Autodesk Fusion 360 part; units mm, degrees
sketch "Base Sketch" plane through (0, 0, 0) normal (0, 0, 1) x (1, 0, 0)
  line L0 (0, 0) -> (106, 0)
  line L1 (106, 0) -> (106, 106)
  line L2 (106, 106) -> (0, 106)
  line L3 (0, 106) -> (0, 0)
  line L4 (19.5, 106) -> (86.5, 106)
  line L5 (86.5, 106) -> (86.5, 0)
  line L6 (86.5, 0) -> (19.5, 0)
  line L7 (19.5, 0) -> (19.5, 106)
  line L8 (21.5, 3) -> (84.5, 3)
  line L9 (84.5, 3) -> (84.5, 104)
  line L10 (84.5, 104) -> (21.5, 104)
  line L11 (21.5, 104) -> (21.5, 3)
  circle A0 centre (23, 7) radius 3
  circle A1 centre (23, 7) radius 0.9
  circle A2 centre (83, 7) radius 0.9
  circle A3 centre (83, 7) radius 3
  circle A4 centre (83, 99) radius 0.9
  circle A5 centre (83, 99) radius 3
  circle A6 centre (23, 99) radius 0.9
  circle A7 centre (23, 99) radius 3
  line L12 (80, 106) -> (80, 104)
  line L13 (52, 106) -> (52, 104)
  line L14 (37, 106) -> (37, 104)
  line L15 (86.5, 5) -> (106, 5)
  line L16 (106, 5) -> (106, 0)
  line L17 (106, 0) -> (86.5, 0)
  line L18 (86.5, 0) -> (86.5, 5)
  line L19 (0, 5) -> (19.5, 5)
  line L20 (19.5, 5) -> (19.5, 0)
  line L21 (19.5, 0) -> (0, 0)
  line L22 (0, 0) -> (0, 5)
  line L23 (86.5, 106) -> (106, 106)
  line L24 (106, 106) -> (106, 98.5)
  line L25 (106, 98.5) -> (86.5, 98.5)
  line L26 (86.5, 98.5) -> (86.5, 106)
  line L27 (0, 106) -> (19.5, 106)
  line L28 (19.5, 106) -> (19.5, 98.5)
  line L29 (19.5, 98.5) -> (0, 98.5)
  line L30 (0, 98.5) -> (0, 106)
  line L31 (106, 76.5) -> (86.5, 76.5)
  line L32 (86.5, 76.5) -> (86.5, 80)
  line L33 (86.5, 80) -> (106, 80)
  line L34 (106, 80) -> (106, 76.5)
  line L35 (0, 76.5) -> (19.5, 76.5)
  line L36 (19.5, 76.5) -> (19.5, 80)
  line L37 (19.5, 80) -> (0, 80)
  line L38 (0, 80) -> (0, 76.5)
  line L39 (63.5, 104) -> (80, 104)
  line L40 (80, 104) -> (80, 81)
  line L41 (36.5, 8) -> (71.5, 8)
  line L42 (71.5, 52) -> (83, 52)
  line L43 (83, 52) -> (83, 9.5)
  line L44 (83, 9.5) -> (71.5, 9.5)
  line L45 (71.5, 9.5) -> (71.5, 52)
  line L46 (62, 106) -> (62, 104)
  line L47 (62, 104) -> (62, 81)
  line L48 (36.5, 80) -> (71.5, 80)
  line L49 (36.5, 80) -> (36.5, 8)
  line L50 (71.5, 8) -> (71.5, 80)
  line L51 (62, 81) -> (80, 81)
  line L52 (36.5, 80) -> (62, 80)
  line L53 (62, 80) -> (62, 82)
  line L54 (62, 82) -> (36.5, 82)
  line L55 (36.5, 82) -> (36.5, 80)
  line L56 (62, 106) -> (60, 106)
  line L57 (60, 106) -> (60, 82)
  line L58 (60, 82) -> (62, 82)
  line L59 (62, 82) -> (62, 106)
  line L60 (80, 81) -> (82, 81)
  line L61 (82, 81) -> (82, 106)
  line L62 (82, 106) -> (80, 106)
  line L63 (80, 106) -> (80, 81)
  line L64 (82, 81) -> (71.5, 81)
  line L65 (71.5, 81) -> (71.5, 79)
  line L66 (71.5, 79) -> (82, 79)
  line L67 (82, 79) -> (82, 81)
  line L68 (71.5, 79) -> (73.5, 79)
  line L69 (73.5, 79) -> (73.5, 52)
  line L70 (73.5, 52) -> (71.5, 52)
  line L71 (71.5, 52) -> (71.5, 79)
  line L72 (36.5, 82) -> (34.5, 82)
  line L73 (34.5, 82) -> (34.5, 6)
  line L74 (34.5, 6) -> (36.5, 6)
  line L75 (36.5, 6) -> (36.5, 82)
  line L76 (36.5, 6) -> (71.5, 6)
  line L77 (71.5, 6) -> (71.5, 8)
  line L78 (71.5, 8) -> (36.5, 8)
  line L79 (36.5, 8) -> (36.5, 6)
  line L80 (71.5, 6) -> (72.5, 6)
  line L81 (72.5, 6) -> (72.5, 52)
  line L82 (72.5, 52) -> (71.5, 52)
  line L83 (71.5, 52) -> (71.5, 6)
  line L84 (62, 81) -> (73.5, 81)
  line L85 (73.5, 81) -> (73.5, 82)
  line L86 (73.5, 82) -> (62, 82)
  line L87 (62, 82) -> (62, 81)
  line L88 (73.5, 81) -> (73.5, 79)
  line L89 (51, 55) -> (59, 55)
  line L90 (59, 55) -> (59, 51)
  line L91 (59, 51) -> (51, 51)
  line L92 (51, 51) -> (51, 55)
  circle A8 centre (60.5, 22.5) radius 2
  circle A9 centre (40, 21.5) radius 1.5
  circle A10 centre (40, 13.5) radius 1.5
  dimension "d1" = 106
  dimension "d2" = 106
  dimension "d4" = 67
  dimension "d5" = 19.5
  dimension "d6" = 63
  dimension "d8" = 2
  dimension "d9" = 3
  dimension "d10" = 6
  dimension "d12" = 6
  dimension "d13" = 6
  dimension "d14" = 6
  dimension "d15" = 23
  dimension "d16" = 23
  dimension "d17" = 23
  dimension "d18" = 23
  dimension "d19" = 7
  dimension "d20" = 7
  dimension "d21" = 7
  dimension "d22" = 7
  dimension "d24" = 2
  dimension "d25" = 6.5
  dimension "d28" = 15
  dimension "d35" = 5
  dimension "d36" = 5
  dimension "d37" = 7.5
  dimension "d38" = 7.5
  dimension "d39" = 3.5
  dimension "d40" = 26
  dimension "d41" = 3.5
  dimension "d42" = 26
  dimension "d45" = 8
  dimension "d48" = 42.5
  dimension "d49" = 9.5
  dimension "d60" = 10
  dimension "d62" = 18
  dimension "d63" = 1.8
  dimension "d64" = 1.8
  dimension "d65" = 1.8
  dimension "d66" = 1.8
  dimension "d68" = 72
  dimension "d69" = 25
  dimension "d70" = 35
  dimension "d71" = 2
  dimension "d72" = 2
  dimension "d73" = 2
  dimension "d74" = 2
  dimension "d75" = 2
  dimension "d76" = 11.5
  dimension "d77" = 2
  dimension "d78" = 2
  dimension "d87" = 1
  dimension "d88" = 25.5
  dimension "d89" = 44
  dimension "d90" = 36.5
  dimension "d94" = 1
  dimension "d95" = 11.5
  dimension "d96" = 8
  dimension "d97" = 4
  dimension "d98" = 25
  dimension "d99" = 14.5
  dimension "d100" = 4
  dimension "d101" = 3
  dimension "d102" = 3
  dimension "d103" = 5.5
  dimension "d104" = 13.5
  dimension "d105" = 3.5
  dimension "d106" = 3.5
  dimension "d107" = 14.5
  dimension "d108" = 24
extrude "Extrude1" add sketch "Base Sketch" against normal blind 9 contours L0 L3 L7 L19 L20 L21 L22 | L0 L2 L4 L5 L6 L7 L8 L9 L10 L11 A0 A3 A5 A7 L14 L18 L20 L26 L28 L32 L36 L61 | L0 L1 L5 L15 L16 L17 L18 | L3 L7 L35 L36 L37 L38 | L1 L5 L31 L32 L33 L34 | L2 L3 L7 L27 L28 L29 L30 | L1 L2 L5 L23 L24 L25 L26 | L2 L4 L10 L12 L61 L62 L63 | A5 L61 | L9 A5 L61 | L11 A7 | L11 A7 | L9 A5 | L11 A0 | L11 A0 | L9 A3 | L9 A3 L43 L44 | A3 L43 L44 makes body 1
extrude "Extrude2" add sketch "Base Sketch" against normal blind 6 contours L2 L4 L10 L13 L14 bodies 1
extrude "Extrude3" add sketch "Base Sketch" against normal blind 5 contours L2 L4 L10 L13 L57 | L2 L4 L10 L46 L56 L57 L59 bodies 1
extrude "Extrude4" add sketch "Base Sketch" against normal blind 2 separate body contours L0 L2 L4 L5 L6 L7 L8 L9 L10 L11 A0 A3 A5 A7 L14 L18 L20 L26 L28 L32 L36 L61 | L2 L4 L10 L13 L14 | L2 L4 L10 L12 L61 L62 L63 | L2 L4 L10 L13 L57 | L8 L9 L10 L11 A0 A3 A7 L44 L54 L57 L72 L73 L74 L76 L80 L81 | L2 L4 L10 L12 L39 L46 L59 L63 | L9 L10 A5 L61 | L2 L4 L10 L46 L56 L57 L59 | A5 L61 | L9 A5 L61 | L10 L47 L54 L57 L58 L59 | L11 A7 | L11 A7 | A5 L40 L60 L61 L63 L64 | L9 A5 | L9 A3 A5 L42 L43 L61 L66 L67 L69 | L47 L48 L52 L53 L54 L55 L58 L75 L87 | L51 L60 L64 L66 L67 L88 | L49 L55 L72 L73 L74 L75 L79 | L11 A0 | L11 A0 | L48 L51 L53 L65 L84 | L50 L51 L64 L65 L66 L68 L84 L88 | L9 A3 | L9 A3 L43 L44 | L42 L50 L66 L68 L69 L70 L71 L82 | A3 L43 L44 | L41 L75 L76 L77 L78 L79 L83 | L44 L50 L77 L80 L81 L83 | A1 | A2 | A4 | A6 makes body 2
chamfer "Chamfer1" distance 8 angle 45 1 edges at (106, 102.25, 0) on bodies 1
chamfer "Chamfer2" distance 8 angle 45 1 edges at (106, 78.25, 0) on bodies 1
chamfer "Chamfer3" distance 8 angle 45 1 edges at (106, 2.5, 0) on bodies 1
chamfer "Chamfer4" distance 8 angle 45 1 edges at (0, 102.25, 0) on bodies 1
chamfer "Chamfer5" distance 8 angle 45 1 edges at (0, 78.25, 0) on bodies 1
chamfer "Chamfer6" distance 8 angle 45 1 edges at (0, 2.5, 0) on bodies 1
extrude "Extrude5" add sketch "Base Sketch" along normal blind 7 contours L47 L48 L52 L53 L54 L55 L58 L75 L87 | L49 L55 L72 L73 L74 L75 L79 | L48 L51 L53 L65 L84 | L50 L51 L64 L65 L66 L68 L84 L88 | L42 L50 L66 L68 L69 L70 L71 L82 | L41 L75 L76 L77 L78 L79 L83 | L44 L50 L77 L80 L81 L83 | L42 L44 L45 L50 L70 L81 L82 L83 bodies 2
extrude "Extrude6" add sketch "Base Sketch" along normal blind 2 from surface at 7 separate body contours L47 L48 L52 L53 L54 L55 L58 L75 L87 | L49 L55 L72 L73 L74 L75 L79 | L48 L51 L53 L65 L84 | L50 L51 L64 L65 L66 L68 L84 L88 | L41 L45 L48 L49 L50 L52 L65 L71 L75 L78 L83 | L42 L50 L66 L68 L69 L70 L71 L82 | L41 L75 L76 L77 L78 L79 L83 | L44 L50 L77 L80 L81 L83 | L42 L44 L45 L50 L70 L81 L82 L83 makes body 3
extrude "Extrude7" add sketch "Base Sketch" along normal blind 5.5 contours L2 L4 L10 L12 L61 L62 L63 | L10 A5 L40 L61 L63 | L2 L4 L10 L46 L56 L57 L59 | A5 L61 | L10 L47 L54 L57 L58 L59 | A5 L40 L60 L61 L63 L64 | L51 L60 L64 L66 L67 L88 bodies 2 1
extrude "Extrude8" add sketch "Base Sketch" along normal blind 2 from surface at 5.5 separate body contours L2 L4 L10 L12 L61 L62 L63 | L2 L4 L10 L12 L39 L46 L59 L63 | L10 A5 L40 L61 L63 | L2 L4 L10 L46 L56 L57 L59 | L10 L39 L40 L47 L51 L59 L63 L64 L85 L86 | A5 L61 | L10 L47 L54 L57 L58 L59 | A5 L40 L60 L61 L63 L64 | L51 L60 L64 L66 L67 L88 makes body 4
extrude "Extrude9" add sketch "Base Sketch" along normal blind 3.5 from surface at 5.5 contours L47 L51 L53 L64 L84 L85 L86 L87 bodies 2 3 4
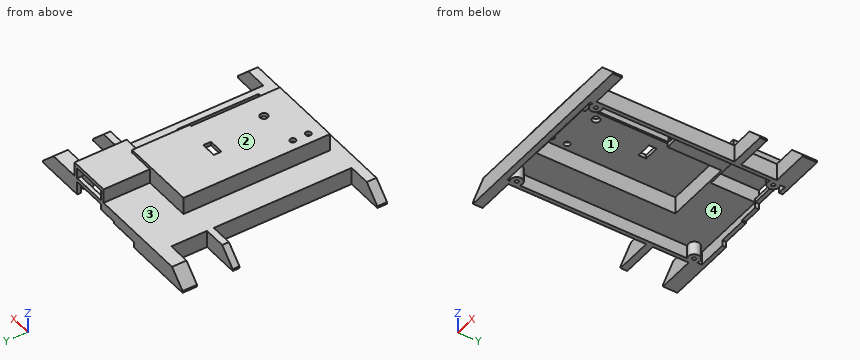
Design review of the part built by this model. Coordinates are the model's own, in mm. Face numbers are marked on the shaded views. A direction names the side the tool comes from. Coordinates: 2 decimals unless noted, no trailing zeros. Write each loop counter-clockwise with the first axis right and the second up, starting at its lowest first coordinate (ties: lowest second). Pieces come first, ordered by that corner, then holes. Notation, with made-up numbers: (-32.75, 58) - (-28.75, 58) arc R26 cw to (-28.75, 74) - close; hole circle Ø9 at (80.5, -40). An arc over 180 degrees is marked (long way). Use one line per item in the form item = value.
Q1. The part is to be moulded in two halves that separate along X. For the marked faces 3 and 4, say which applies: +X half, -X half, draft (parallel to the pull), parting line (faces both ways), or undercut.
Taken from the geometry:
face_3 = draft
face_4 = undercut
Q2. For probe 1 along Y at (x, z) = (98.5, -3.5); probe 2 along Y at (x, z) = (23, -6.5); probe 3 along Y at (x, z) = (41, -5.75), list the stretches that pass through material, from the lowest coordinate up.
Taken from the geometry:
probe_1 = 0 to 5, 76.5 to 80, 98.5 to 106
probe_2 = 0 to 3, 4 to 6.1, 7.9 to 10, 96 to 98.1, 99.9 to 102, 104 to 106
probe_3 = 0 to 3, 104 to 106
Q3. Consider section D-D (z = 2.75). Write out the cut boundary in (x, y), plus the area to 4 significant figures.
Taken from the geometry:
outline = (34.5, 6) - (72.5, 6) - (72.5, 52) - (73.5, 52) - (73.5, 79) - (82, 79) - (82, 106) - (80, 106) - (80, 81) - (62, 81) - (62, 106) - (60, 106) - (60, 82) - (34.5, 82) - close; hole (36.5, 8) - (71.5, 8) - (71.5, 80) - (36.5, 80) - close
area = 501.5 mm^2
Q4. Machinability: for the marked faces 1 and 2, which of the approach directions +Z, -Z, +X, -X, +Y, -Y give a long, thin tool a straight path to every point of the face, cutting with its end or side? Answer none if there is none.
Taken from the geometry:
face_1 = -Z
face_2 = +Z, +X, -X, +Y, -Y
Q5. Consider section B-B (y = 13.5). Write out the cut boundary in (x, z).
Taken from the geometry:
outline = (19.5, -9) - (21.5, -9) - (21.5, -2) - (36.5, -2) - (36.5, 7) - (38.5, 7) - (38.5, 9) - (34.5, 9) - (34.5, 0) - (19.5, 0) - close; (41.5, 7) - (71.5, 7) - (71.5, 0) - (72.5, 0) - (72.5, 9) - (41.5, 9) - close; (83, -2) - (84.5, -2) - (84.5, -9) - (86.5, -9) - (86.5, 0) - (83, 0) - close
Q6. Consider section A-A (x = 66). Write out the cut boundary in (y, z).
Taken from the geometry:
outline = (0, -9) - (3, -9) - (3, -2) - (8, -2) - (8, 7) - (80, 7) - (80, -2) - (81, -2) - (81, 5.5) - (106, 5.5) - (106, 7.5) - (82, 7.5) - (82, 9) - (6, 9) - (6, 0) - (0, 0) - close; (104, -2) - (106, -2) - (106, 0) - (104, 0) - close
Q7. Insertion check: pin 1 Ø10 at (y, z) = (60.5, 4) entering from +X; pin 2 Ø11 at (x, y) = (67, 92.5) entering from +Z; pin 3 Ø2.5 at (x, y) = (23, 7) entering from +Z. Each pin has a flat end and moves straight along its axis. Give the tip position at first contact, or say it passes through.
Taken from the geometry:
pin_1 = 86.5
pin_2 = 7.5
pin_3 = 0
Q8. Consider section C-C (x = 93.5). Write out the cut boundary in (y, z), plus the area to 3 significant figures.
Taken from the geometry:
outline = (0, -9) - (5, -9) - (5, 0) - (0, 0) - close; (76.5, -9) - (80, -9) - (80, 0) - (76.5, 0) - close; (98.5, -9) - (106, -9) - (106, 0) - (98.5, 0) - close
area = 144 mm^2
